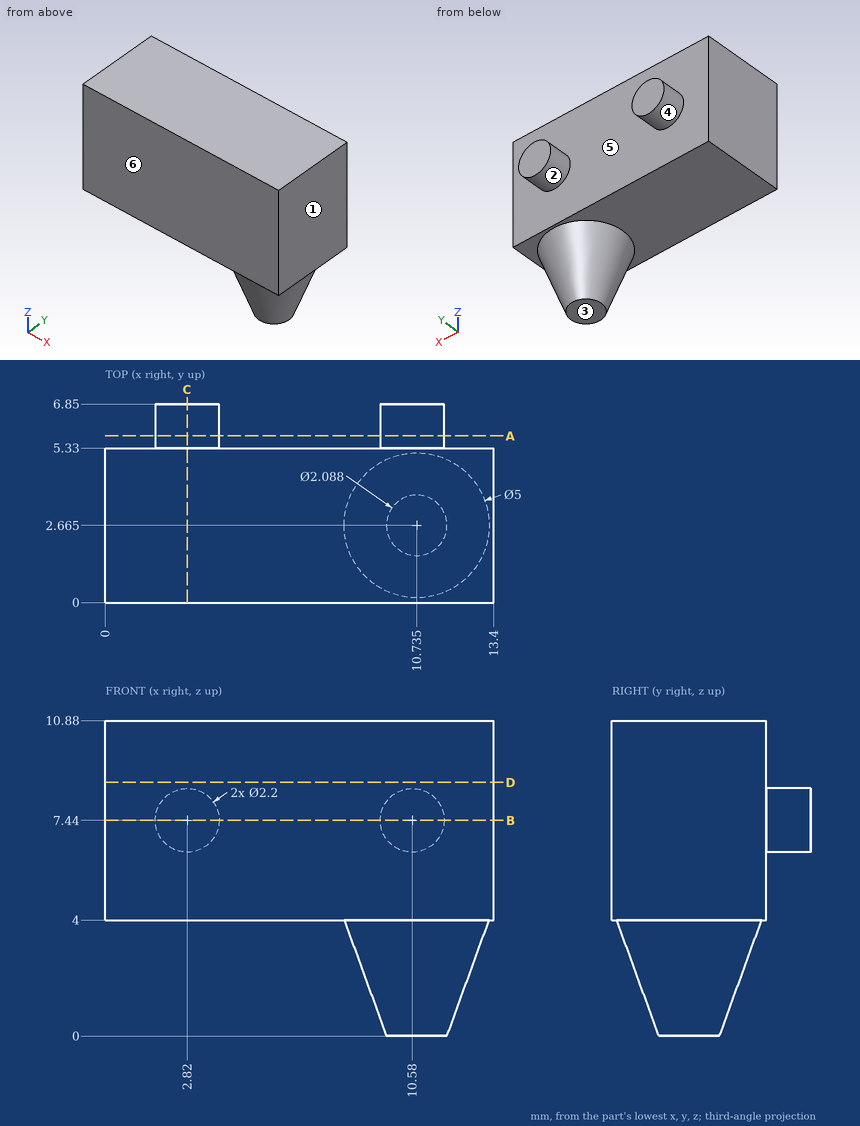
Here's the drawing with two shaded views (mm, measured from the low corner). I have some questions. A direction names the side the tool comes from. Coordinates: 2 decimals unless noted, no trailing zeros. Loops run counter-clockwise (first coordinate to the right, second up) from the corner with the lowest first, then second, coordinate; pieces in that order, holes last. Notation, with made-up numbers: M -20,30 L 7,30 A8 cw 7,40 Z; hole C 14,-40 d1. An arc over 180 degrees is marked long. Put each result on its own line as item: value. Start each with the question number.
(1) Imagine slicing it at C-C on x = 2.82. List the corners of the cut face in (y, z) for me, and give its area (3 significant figures).
(2) Which directions (+Z, -Z, +X, -X, +Y, -Y) give clear straight access to the entire face, cutting with the end or side of a thin tool? Please do the marked faces 5 and 6.
(3) Imagine slicing it at D-D on z = 8.75. List the corners of the cut face in (x, y) for me.
(4) Imagine slicing it at A-A on y = 5.75. List the corners of the cut face in (x, z) for me.
(5) Will this pin go through, and if not, where does the flat tip stop? pin 1 Ø3.5 at (x, z) = (6, 7.5) entering from +Y.
(6) We'd pull the mould along X, two halves only. Please class the marked faces 1, 2, 3 and 4: +X half, -X half, draft (parallel to the pull), parting line (faces both ways), or undercut.
(7) I need wall thicknesses on probe 1 along Z at (x, y) = (7.5, 3.25); probe 2 along Y at (x, z) = (13, 4.75); probe 3 along Z at (x, y) = (9.75, 4.5) (1 decimal). Which ranges of each line are inside material? Lowest first, please.
(8) Imagine slicing it at B-B on z = 7.44. List the corners of the cut face in (x, y) for me, and give its area (3 significant figures).
Worked answers:
1. outline: M 0,4 L 5.33,4 L 5.33,6.34 L 6.85,6.34 L 6.85,8.54 L 5.33,8.54 L 5.33,10.88 L 0,10.88 Z
1. area: 40.0 mm2
2. face 5: +Y
2. face 6: +Z, -Z, +X, -X, -Y
3. outline: M 0,0 L 13.4,0 L 13.4,5.33 L 0,5.33 Z
4. outline: C 2.82,7.44 d2.2; C 10.58,7.44 d2.2
5. pin 1: stops at y = 5.33
6. face 1: +X half
6. face 2: undercut
6. face 3: draft
6. face 4: undercut
7. probe 1: z = 4 to 10.88
7. probe 2: y = 0 to 5.33
7. probe 3: z = 2.9 to 10.9
8. outline: M 0,0 L 13.4,0 L 13.4,5.33 L 11.68,5.33 L 11.68,6.85 L 9.48,6.85 L 9.48,5.33 L 3.92,5.33 L 3.92,6.85 L 1.72,6.85 L 1.72,5.33 L 0,5.33 Z
8. area: 78.1 mm2
